For this review, take the finished solid that the model builds, in its own axes (mm). A direction names the side the tool comes from. Round coordinates to 2 decimals unless told otherwise and drop trailing zeros. Order: outer loops, then holes, each group sorted by start corner. A loop starts at its lowest first (then second) coordinate and runs counter-clockwise, first axis right, second up. Notation, with made-up numbers: (25.5, -16) -> (84.5, -16) arc R11 ccw to (84.5, -10) -> close; hole circle Ø11 at (71.25, 16.5). An arc over 180 degrees is marked (long way). Use a Markdown table: item, result. Add a question column.
1) Draft analysis for pull direction Y (two halves, no side actions). For faces 4 (the face through (25.4, 0, 0)), 5 (the face through (12.38, -0.31, 1.39)), 6 (the face through (-2.154, -0.587, 1.036)), state which applies: pulls with the +Y half, pulls with the -Y half, needs draft (parallel to the pull), parting line crosses it, or undercut.
2) Clearance check with a flat-ended pin moving along its axis: P1, Ø2, axis at x = 4, z = 0.5, coming from the +Y side. State where the tip first meets the part, or that it passes through.
3) Consider section A-A (x = 15.25). State the section outline as (y, z) points.
4) Machinability: for faces 1 (the face through (0, 2, 0)), 2 (the face through (-2.845, -1, 1)), 3 (the face through (-2.15, -0.6, -1.03)), which of the approach directions +Z, -Z, +X, -X, +Y, -Y give a long, thin tool a straight path to every point of the face, cutting with its end or side? Answer none if there is none.
5) Wall thickness on line 1 along X through (y, z) = (0.7, -2); line 2 along Z through (x, y) = (17.75, 0); line 3 along Y through (x, z) = (3.25, -0.8): over which ranges is each line inside the solid? List them lowest first. Write a range as [from, to].
Autodesk Inventor part; units mm, degrees
ref_plane "Work Plane1" through (29, 0, 0) normal (0, -1, 0) x (1, 0, 0)
ref_plane "YZ Plane" through (0, 0, 0) normal (1, 0, 0) x (0, 1, 0)
ref_plane "XZ Plane" through (0, 0, 0) normal (0, 1, 0) x (-1, 0, 0)
sketch "Sketch1" plane through (0, 0, 0) normal (0, 0, 1) x (1, 0, 0)
  line L0 (-0.7556, 0) -> (25.4, 0)
  line L1 (25.4, 0) -> (25.4, 1.4224)
  line L2 (25.4, 1.4224) -> (6.35, 1.4224)
  line L3 (6.35, 1.4224) -> (5.0799, 1.4224)
  line L4 (5.0799, 1.4224) -> (0, 1.4224)
  line L5 (0, 1.4224) -> (0, 2.3241)
  line L6 (0, 2.3241) -> (-2.8448, 2.3241)
  line L7 (-2.8448, 2.3241) -> (-2.8448, 1.3748)
  line L8 (-2.8448, 1.3748) -> (-1.5494, 1.3748)
  line L9 (-1.5494, 1.3748) -> (-0.7556, 0)
  line L10 (-8.4938, 0) -> (31.049, 0)
  line L11 (0, -0.4648) -> (0, 2.7889)
  line L12 (6.35, 1.4224) -> (0, 1.4224) construction
  dimension "d1" = 19.05
  dimension "d2" = 1.2701
  dimension "d3" = 2.8448
  dimension "d4" = 1.2954
  dimension "d5" = 60
  dimension "d6" = 2.8448
  dimension "d7" = 2.8448
  dimension "d8" = 2.7496
  dimension "d9" = 4.6482
  dimension "d26" = 25.4
revolve "Body" add sketch "Sketch1" angle 360 about axis through (-0.7556, 0, 0) along (1, 0, 0)
sketch "Sketch2" plane through (-2.8448, 0, 0) normal (-1, 0, 0) x (0, 0, 1)
  circle A0 centre (0, 0) radius 1.3748
  line L0 (0, -3.2537) -> (0, 3.2537)
  line L1 (-3.2537, 0) -> (3.2537, 0)
  line L2 (1.3748, 0) -> (0.6874, -1.1906)
  line L3 (0.6874, -1.1906) -> (-0.6874, -1.1906)
  line L4 (-0.6874, -1.1906) -> (-1.3748, 0)
  line L5 (-1.3748, 0) -> (-0.6874, 1.1906)
  line L6 (-0.6874, 1.1906) -> (0.6874, 1.1906)
  line L7 (0.6874, 1.1906) -> (1.3748, 0)
  point P0 (0, 0)
extrude "Slot" add sketch "Sketch2" against normal up to next contours L7 A0 | A0 L2 | L6 L0 A0 | A0 L0 L3 | L0 L6 A0 | A0 L3 L0 | L4 A0 | A0 L5
fillet "Fillet1" radius 0.2286 1 edges at (-2.8448, -2.3241, 0)
thread "Thread"
chamfer "Chamfer1" distance 0.3895 distance2 0.3896 1 edges at (25.4, -1.4224, 0) measured on face at (25.4, 0.2736, 0.8712)
ref_plane "Work Plane1" through (29, 0, 0) normal (0, -1, 0) x (1, 0, 0)
fillet "Fillet2" radius 0.1 1 edges at (0, -1.4224, 0)
equation "\"d1\" = GEL"
equation "\"d3\" = KOH"
equation "\"d4\" = INTI"
equation "\"d6\" = GD"
equation "\"d7\" = BDM"
equation "\"d8\" = 1.1547 * SW"
equation "\"d9\" = KOD"
equation "\"d26\" = NLG"
equation "\"d30\" = R"
equation "\"d17\" = RR"
equation "\"d13\" = GEL"
equation "\"d15\" = -0.5 * SPD + 0.5 * GD"
equation "\"d16\" = GUL"
equation "\"GD\" = NND"
equation "\"NLG\" = 25.4"
equation "\"GEL\" = 19.05"
equation "\"KOD\" = 4.6482"
equation "\"KOH\" = NND"
equation "\"INTI\" = 1.2954"
equation "\"GAL\" = 1.27"
equation "\"GUL\" = 0.38964"
equation "\"BDM\" = NND"
equation "\"SW\" = 2.38125"
equation "\"RR\" = 0.2286"
equation "\"SPD\" = GD1"
equation "\"R\" = 0.1"
equation "\"PHH\" = 0.1 * NND"
equation "\"THREADDIA\" = 2.8448"
equation "\"FAWI\" = 45deg"
equation "\"NND\" = 2.8448"
equation "\"E0\" = 1.155 * SW"
equation "\"FAWI1\" = 30deg"
equation "\"TOA\" = 30deg"
equation "\"GD1\" = 2.06573"
properties part number "Unbrako - 4 x 1" material "Steel, Mild"
Results list:
| question | item | result |
|---|---|---|
| 1 | face 4 | needs draft |
| 1 | face 5 | parting line crosses it |
| 1 | face 6 | undercut |
| 2 | P1 | y = 1.42 |
| 3 | outline | circle Ø2.84 at (0, 0) |
| 4 | face 1 | +X |
| 4 | face 2 | +Z, -Z, -X, +Y, -Y |
| 4 | face 3 | -X |
| 5 | line 1 | [-2.84, 0] |
| 5 | line 2 | [-1.42, 1.42] |
| 5 | line 3 | [-1.18, 1.18] |
